Geometry check sheet. Reference: drawing and pictorial views, mm from the part's lowest x, y, z. A direction names the side the tool comes from. Coordinates: 2 decimals unless noted, no trailing zeros. Loops run counter-clockwise (first coordinate to the right, second up) from the corner with the lowest first, then second, coordinate; pieces in that order, holes last. Notation, with made-up numbers: (-39, 42) -> (4, 42) arc R8 cw to (4, 50) -> close; hole circle Ø4 at (23, 43). An arc over 180 degrees is marked (long way). Answer as a JSON object with one key per item and string values. Group by question number.
Q1. Cross-section at B-B on y = 14.5. Record the boundary of the cut face in (x, z).
Q2. Scan lines: L1, parallel to Z at x = 3, y = 138.5; L2, parallel to X at y = 119.5, z = 20; L3, parallel to Z at x = 16, y = 146.5. Record each from-to range of solid material in increasing order.
Q3. Cross-section at C-C on y = 45.5. Record the boundary of the cut face in (x, z), and give its area (3 significant figures).
Q4. Cross-section at D-D on z = 25.5. Record the boundary of the cut face in (x, y), and give its area (3 significant figures).
Q5. Gauge pin test, flat end, axial feed: pin 1 Ø1.5 at (y, z) = (77, 27) entering from -X. Record the tip position at first contact, or that the pin passes through.
Q6. Release check for a two-part mould opening along Z. For the marked faces 3, 4 and 5 record: released by +Z, released by -Z, zero draft, split by the parting line, or undercut.
Q7. Cross-section at A-A on x = 4. Record the boundary of the cut face in (y, z).
Q8. Set-up check for the marked faces 1 and 2: record each of +Z, -Z, +X, -X, +Y, -Y from which the full face is reachable in a straight line by a thin tool's end or side.
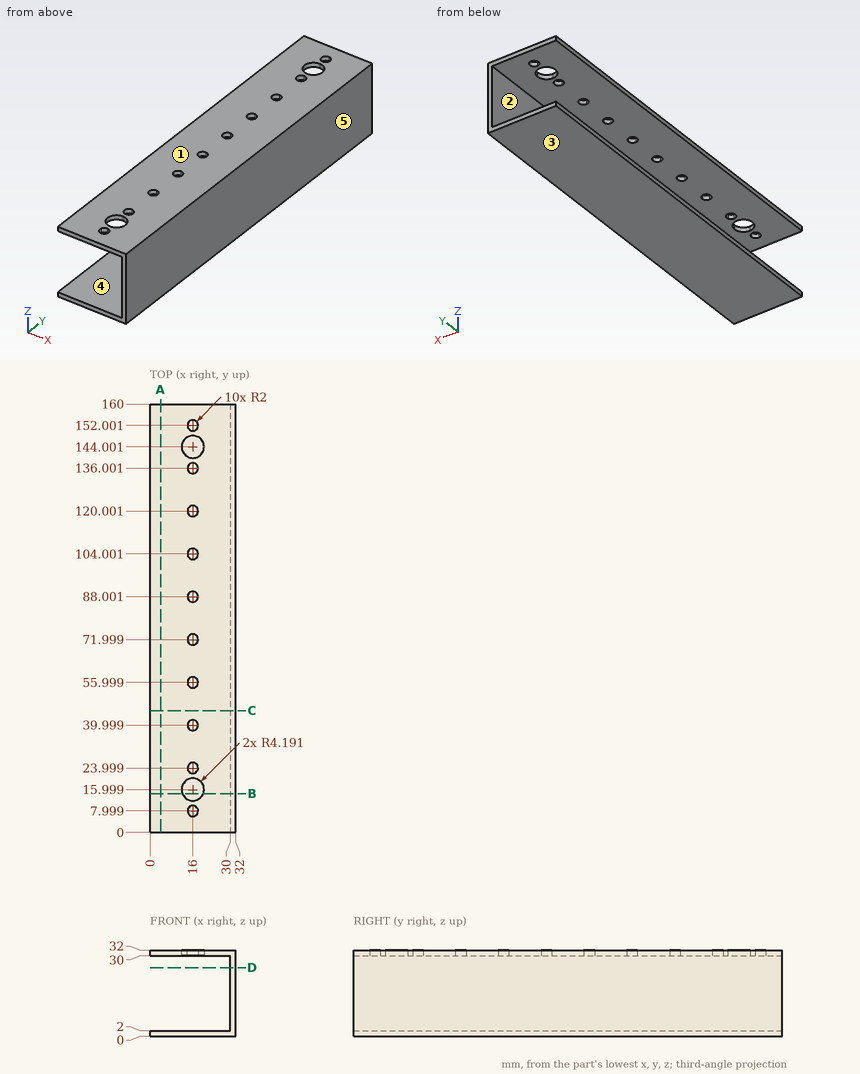
Computed values:
{
 "1": {"outline": "(0, 0) -> (32, 0) -> (32, 32) -> (19.91, 32) -> (19.91, 30) -> (30, 30) -> (30, 2) -> (0, 2) -> close; (0, 30) -> (12.09, 30) -> (12.09, 32) -> (0, 32) -> close"},
 "2": {"L1": "z = 0 to 2, 30 to 32", "L2": "x = 30 to 32", "L3": "z = 0 to 2"},
 "3": {"outline": "(0, 0) -> (32, 0) -> (32, 32) -> (0, 32) -> (0, 30) -> (30, 30) -> (30, 2) -> (0, 2) -> close", "area": "184 mm²"},
 "4": {"outline": "(30, 0) -> (32, 0) -> (32, 160) -> (30, 160) -> close", "area": "320 mm²"},
 "5": {"pin 1": "stops at x = 30"},
 "6": {"face 3": "released by -Z", "face 4": "undercut", "face 5": "zero draft"},
 "7": {"outline": "(0, 0) -> (160, 0) -> (160, 2) -> (0, 2) -> close; (0, 30) -> (160, 30) -> (160, 32) -> (0, 32) -> close"},
 "8": {"face 1": "+Z, +X, -X, +Y, -Y", "face 2": "-X, +Y, -Y"}
}
